For this review, take the finished solid that the model builds, in its own axes (mm). A direction names the side the tool comes from. Give positions to 0.01 mm unless a question says otherwise; leave off trailing zeros. Order: outer loops, then holes, each group sorted by start corner. A loop starts at its lowest first (then second) coordinate and runs counter-clockwise, first axis right, second up. Notation, with made-up numbers: (7, -39.5) -> (51, -39.5) arc R5 ccw to (51, -35.5) -> close; hole circle Ø9 at (-37.75, -28.5). An arc over 180 degrees is marked (long way). One line per item, written item: value. Start each with the question number.
Autodesk Inventor part; units mm, degrees
ref_plane "YZ Plane" through (0, 0, 0) normal (1, 0, 0) x (0, 1, 0)
ref_plane "XZ Plane" through (0, 0, 0) normal (0, 1, 0) x (-1, 0, 0)
ref_plane "XY Plane" through (0, 0, 0) normal (0, 0, 1) x (1, 0, 0)
sketch "Szkic1" plane through (0, 0, 0) normal (0, 1, 0) x (-1, 0, 0)
  circle A0 centre (0, 0) radius 3.5
  line L0 (0.7217, 1.25) -> (1.4434, 0)
  line L1 (1.4434, 0) -> (0.7217, -1.25)
  line L2 (0.7217, -1.25) -> (-0.7217, -1.25)
  line L3 (-0.7217, -1.25) -> (-1.4434, 0)
  line L4 (-1.4434, 0) -> (-0.7217, 1.25)
  line L5 (-0.7217, 1.25) -> (0.7217, 1.25)
  circle A1 centre (0, 0) radius 1.5
  dimension "d0" = 7
  dimension "d1" = 2.5
  dimension "d2" = 3
extrude "Wyciągnięcie proste1" add sketch "Szkic1" along normal blind 1.5 contours A0 | L0 L1 L2 L3 L4 L5 | A1
extrude "Wyciągnięcie proste2" add sketch "Szkic1" against normal blind 1.5 contours A0 | A1
sketch "Szkic2" plane through (0, 1.5, 0) normal (0, 1, 0) x (1, 0, 0)
  circle A0 centre (0, 0) radius 1.5
  dimension "d7" = 3
extrude "Wyciągnięcie proste3" add sketch "Szkic2" along normal blind 30
thread "Gwint1"
properties part number "M3x30"
Q1. Take a section at D-D (x = 2.5). State the section outline as (y, z) points.
Q2. For faces 1 (the flat face through (-1.08, -0.74, 0.63)), 2 (the flat face through (0, 1.5, -2)), 3 (the flat face through (0, 31.5, 0)), list the 3-axis set-ups (+Z, -Z, +X, -X, +Y, -Y) from which the entire face can be reached by the end or side of a thin tool; tool diameter is ignored.
Q3. For pin 1 Ø1.5 at (x, y) = (0, 23.5) entering from -Z; pin 2 Ø1 at (x, y) = (-1.5, 8) entering from +Z; pin 3 Ø0.8 at (x, z) = (0, 0.5) entering from -Y; pin 4 Ø3 at (x, z) = (0.5, -1) entering from -Y, all flat-tipped, find the tip position at first contact; note any pin that passes through.
Q4. For line 1 along Y through (x, z) = (-3, -1.75); line 2 along Y through (x, z) = (-0.5, -1); line 3 along Z through (x, y) = (-1.25, 4), list the stretches that pass through material, from the lowest coordinate up.
Q5. Take a section at C-C (z = -2). State the section outline as (x, y) points, and give its area (3 significant figures).
Q6. Take a section at B-B (y = 26.5). State the section outline as (x, z) points, and give its area (3 significant figures).
Q7. Mouldability with a two-part tool opening along X and no side actions: class faces 4 (the flat face through (-1.088, -0.74, -0.616)), 5 (the cylindrical face through (-1.5, 16.29, 0.07)), 6 (the flat face through (0, -1.5, -2)) as pulls with the +X half, pulls with the -X half, needs draft (parallel to the pull), parting line crosses it, or undercut.
Q8. Take a section at A-A (x = 0). State the section outline as (y, z) points.
Answers below:
1. outline: (-1.5, -2.45) -> (1.5, -2.45) -> (1.5, 2.45) -> (-1.5, 2.45) -> close
2. face 1: -Y
2. face 2: +Y
2. face 3: +Z, -Z, +X, -X, +Y
3. pin 1: stops at z = -1.5
3. pin 2: stops at z = 1.12
3. pin 3: stops at y = 0
3. pin 4: stops at y = -1.5
4. line 1: y = -1.5 to 1.5
4. line 2: y = 0 to 31.5
4. line 3: z = -0.83 to 0.83
5. outline: (-2.87, -1.5) -> (2.87, -1.5) -> (2.87, 1.5) -> (-2.87, 1.5) -> close
5. area: 17.2 mm²
6. outline: circle Ø3 at (0, 0)
6. area: 7.07 mm²
7. face 4: undercut
7. face 5: parting line crosses it
7. face 6: needs draft
8. outline: (-1.5, -3.5) -> (1.5, -3.5) -> (1.5, -1.5) -> (31.5, -1.5) -> (31.5, 1.5) -> (1.5, 1.5) -> (1.5, 3.5) -> (-1.5, 3.5) -> (-1.5, 1.25) -> (0, 1.25) -> (0, -1.25) -> (-1.5, -1.25) -> close
